Work out the finished part from the listing and answer in its coordinate system (mm). A direction names the side the tool comes from. Coordinates: 2 decimals unless noted, no trailing zeros. Order: outer loops, then holes, each group sorted by start corner. A loop starts at its lowest first (then second) coordinate and runs counter-clockwise, first axis right, second up. Notation, with made-up numbers: M 30.5,73 L 86.5,73 A17 cw 86.5,82 Z; hole C 51,84 d4. An arc over 180 degrees is marked long. Write item = value, one per line. Start each with the question number.
Q1. Each of these flat-tipped pins is pushed along its axis until it touches: P1, Ø4, axis at x = -3, z = 1.5, coming from the +Y side; P2, Ø6, axis at x = 2.5, y = 6.5, coming from the +Z side; P3, Ø2, axis at x = -4, z = -12, coming from the -Y side. Where does it stop, or does it pass through?
Q2. Determine the mould class of faces 1 (the flat face through (4, 18, -16.25)), 2 (the flat face through (-6.25, 12, 0)), 3 (the cylindrical face through (0, 17.5, 13.7)) for opening direction Z: released by +Z, released by -Z, zero draft, split by the parting line, or undercut.
Q3. Find section A-A on z = 15.2. Give the vertices of the cut face in (x, y).
Q4. A tool of negligible diameter and unlimited length cuts with its end or side. For faces 4 (the flat face through (-5, 2, -10)), 5 (the flat face through (3.95, 1.2, -9.6)), 6 (the cylindrical face through (0.751, 28.679, -2.865)), 7 (the flat face through (-5, 24, -10)), 8 (the flat face through (0, 26, 10.129)), from which of +Z, -Z, +X, -X, +Y, -Y can it reach the whole face along a straight path? Write none if from no direction.
Q5. Find section B-B on y = 9. Give the vertices of the cut face in (x, z).
Q6. Find section D-D on y = 18. Give the vertices of the cut face in (x, z).
Q7. Find section C-C on z = 5. Give the vertices of the cut face in (x, y).
Q8. Straight lines are drawn through the part: line 1 along X through (y, z) = (17.05, 15.2); line 2 along Y through (x, z) = (-5.5, 6); line 3 along Z through (x, y) = (0.75, 23). For each, find the intervals that lie inside material, in ascending order.
```python
from build123d import *

# Parameters (mm, degrees)
SKETCH1_W               = 12.5
SKETCH1_H               = 23
BOSS_EXTRUDE1_DEPTH     = 24
BOSS_EXTRUDE2_DEPTH     = 3.2
SKETCH3_R               = 2.5
SKETCH3_R_2             = 0.5
BOSS_EXTRUDE3_DEPTH     = 3
SKETCH4_W               = 12.5
SKETCH4_H               = 2.5
BOSS_EXTRUDE4_DEPTH     = 4.75
SKETCH5_W               = 12.5
SKETCH5_H               = 2.5
BOSS_EXTRUDE5_DEPTH     = 4.75
CUT_EXTRUDE1_REACH      = 27.55
SKETCH6_R               = 1.5
CUT_EXTRUDE2_REACH      = 27.697
SKETCH8_R               = 1.5
CUT_EXTRUDE4_DEPTH      = 37.501404083
CUT_EXTRUDE6_DEPTH      = 37.501404083
CUT_EXTRUDE6_DEPTH_BACK = 2.3
CUT_EXTRUDE7_DEPTH      = 37.501404083
CUT_EXTRUDE7_DEPTH_BACK = 2.3
FILLET1_R               = 0.5


with BuildPart() as part:
    # Sketch1 → Boss-Extrude1 (new body)
    with BuildSketch(Plane(origin=(0, 0, 0), x_dir=(1, 0, 0), z_dir=(0, 1, 0))):
        Rectangle(SKETCH1_W, SKETCH1_H)
    extrude(amount=BOSS_EXTRUDE1_DEPTH)

    # Sketch2 → Boss-Extrude2 (add)
    with BuildSketch(Plane(origin=(0, 24, 0), x_dir=(1, 0, 0), z_dir=(0, 1, 0))):
        with BuildLine():
            Line((-5.757621024, 2.818477812), (-5.757621024, -10.12881992))
            Line((-5.757621024, -10.12881992), (5.781688552, -10.12881992))
            Line((5.781688552, -10.12881992), (5.781688552, 2.876273501))
            ThreePointArc((5.781688552, 2.876273501), (-0.031303305, 11.499921608), (-5.757621024, 2.818477812))
        make_face()
    extrude(amount=BOSS_EXTRUDE2_DEPTH)

    # Sketch3 → Boss-Extrude3 (add)
    with BuildSketch(Plane(origin=(0, 27.2, 0), x_dir=(1, 0, 0), z_dir=(0, 1, 0))):
        with Locations(Location((0, 5.25, 0), (0, 0, 270))):
            Circle(SKETCH3_R)
        with Locations(Location((0, 5.25, 0), (0, 0, 270))):
            Circle(SKETCH3_R_2, mode=Mode.SUBTRACT)
    extrude(amount=BOSS_EXTRUDE3_DEPTH)

    # Sketch4 → Boss-Extrude4 (add)
    with BuildSketch(Plane(origin=(0, 0, -11.5), x_dir=(-1, 0, 0), z_dir=(0, 0, -1))):
        with Locations((0, 17.65)):
            Rectangle(SKETCH4_W, SKETCH4_H)
    extrude(amount=BOSS_EXTRUDE4_DEPTH)

    # Sketch5 → Boss-Extrude5 (add)
    with BuildSketch(Plane.XY.offset(11.5)):
        with Locations((0, 17.45)):
            Rectangle(SKETCH5_W, SKETCH5_H)
    extrude(amount=BOSS_EXTRUDE5_DEPTH)

    # Sketch6 → Cut-Extrude1 (cut, up to next)
    with BuildSketch(Plane(origin=(0, 18.7, 0), x_dir=(1, 0, 0), z_dir=(0, 1, 0)), mode=Mode.PRIVATE) as cut_extrude1_sk1:
        with Locations((0, -15.2)):
            Circle(SKETCH6_R)
    cut_extrude1_tool1 = extrude(cut_extrude1_sk1.sketch, amount=-CUT_EXTRUDE1_REACH, mode=Mode.PRIVATE) & part.part
    add(cut_extrude1_tool1.solids().sort_by_distance((0, 18.7, 15.2))[0], mode=Mode.SUBTRACT)

    # Sketch8 → Cut-Extrude2 (cut, up to next)
    with BuildSketch(Plane(origin=(0, 18.9, 0), x_dir=(1, 0, 0), z_dir=(0, 1, 0)), mode=Mode.PRIVATE) as cut_extrude2_sk1:
        with Locations((0, 15.2)):
            Circle(SKETCH8_R)
    cut_extrude2_tool1 = extrude(cut_extrude2_sk1.sketch, amount=-CUT_EXTRUDE2_REACH, mode=Mode.PRIVATE) & part.part
    add(cut_extrude2_tool1.solids().sort_by_distance((0, 18.9, -15.2))[0], mode=Mode.SUBTRACT)

    # Sketch9 → Cut-Extrude4 (cut, through all)
    with BuildSketch(Plane(origin=(6.25, 0, 0), x_dir=(0, 0, -1), z_dir=(1, 0, 0))):
        Polygon((11.5, 2), (8.5, 0), (11.5, 0), align=None)
    extrude(amount=-CUT_EXTRUDE4_DEPTH, mode=Mode.SUBTRACT)

    # Sketch10 → Cut-Extrude6 (cut, two sides: drawn at the far end of the back side and taken through both)
    with BuildSketch(Plane(origin=(6.25, 0, 0), x_dir=(0, 0, -1), z_dir=(1, 0, 0)).offset(-CUT_EXTRUDE6_DEPTH_BACK)):
        Polygon((100.627808007, 2), (11.5, 2), (8.5, 2), (8.5, 0), (8.5, -89.127808007), (133.856074627, -215.859489897), (225.983882634, -124.73168189), align=None)
    extrude(amount=CUT_EXTRUDE6_DEPTH + CUT_EXTRUDE6_DEPTH_BACK, mode=Mode.SUBTRACT)

    # Sketch11 → Cut-Extrude7 (cut, two sides: drawn at the far end of the back side and taken through both)
    with BuildSketch(Plane.ZY.offset(6.25).offset(-CUT_EXTRUDE7_DEPTH_BACK)):
        Polygon((-100.627808007, 2), (-11.5, 2), (-8.5, 2), (-8.5, 0), (-8.5, -89.127808007), (-133.856074627, -215.859489897), (-225.983882634, -124.73168189), align=None)
    extrude(amount=CUT_EXTRUDE7_DEPTH + CUT_EXTRUDE7_DEPTH_BACK, mode=Mode.SUBTRACT)

    # Fillet1
    fillet1_edges = [part.edges().sort_by_distance(p)[0] for p in [
        (-6.25, 9.2, -11.5),
        (6.25, 9.2, -11.5),
        (6.25, 0, 1.5),
        (6.25, 8.1, 11.5),
        (-6.25, 8.1, 11.5),
        (0, 0, 11.5),
        (-6.25, 21.45, -11.5),
        (6.25, 21.45, -11.5),
        (6.25, 21.35, 11.5),
        (-6.25, 21.35, 11.5),
        (-6.25, 0, 1.5),
    ]]
    fillet(fillet1_edges, radius=FILLET1_R)


solid = part.part
```
Findings below:
q1.P1 = 27.2
q1.P2 = 11.5
q1.P3 = 1.67
q2.face_1 = released by -Z
q2.face_2 = zero draft
q2.face_3 = undercut
q3.outline = M -6.25,16.2 L -1.5,16.2 L -1.5,18.7 L -6.25,18.7 Z; M 1.5,16.2 L 6.25,16.2 L 6.25,18.7 L 1.5,18.7 Z
q4.face_4 = -Z, -X, -Y
q4.face_5 = -Z, +X, -Y
q4.face_6 = +Y
q4.face_7 = -Z, -X, +Y
q4.face_8 = +Z, +X, -X, +Y
q5.outline = M -6.25,-11 A0.5 ccw -5.75,-11.5 L 5.75,-11.5 A0.5 ccw 6.25,-11 L 6.25,11 A0.5 ccw 5.75,11.5 L -5.75,11.5 A0.5 ccw -6.25,11 Z
q6.outline = M -6.25,-16.25 L -1.07,-16.25 A1.5 cw long 1.07,-16.25 L 6.25,-16.25 L 6.25,16.25 L 1.07,16.25 A1.5 cw long -1.07,16.25 L -6.25,16.25 Z
q7.outline = M -6.25,0.5 A0.5 ccw -5.75,0 L 5.75,0 A0.5 ccw 6.25,0.5 L 6.25,24 L 5.78,24 L 5.78,27.2 L -5.76,27.2 L -5.76,24 L -6.25,24 Z
q8.line_1 = -6.25 to -1.5, 1.5 to 6.25
q8.line_2 = 0 to 27.2
q8.line_3 = -11.5 to 11.5
